Input: dimensioned drawing with shaded views. Units: mm. Origin: part minimum x, y, z. Round coordinates to 2 decimals unless told otherwise and drop trailing zeros. Order: outer loops, then holes, each group sorted by start corner. A loop starts at its lowest first (then second) coordinate and runs counter-clockwise, first axis right, second up. Notation, with made-up numbers: (-8.5, 65) -> (27.5, 65) arc R25 ccw to (27.5, 92) -> close; hole circle Ø2 at (52, 88). An arc over 180 degrees is marked (long way). Use a Markdown table: item, result. Add a question column.
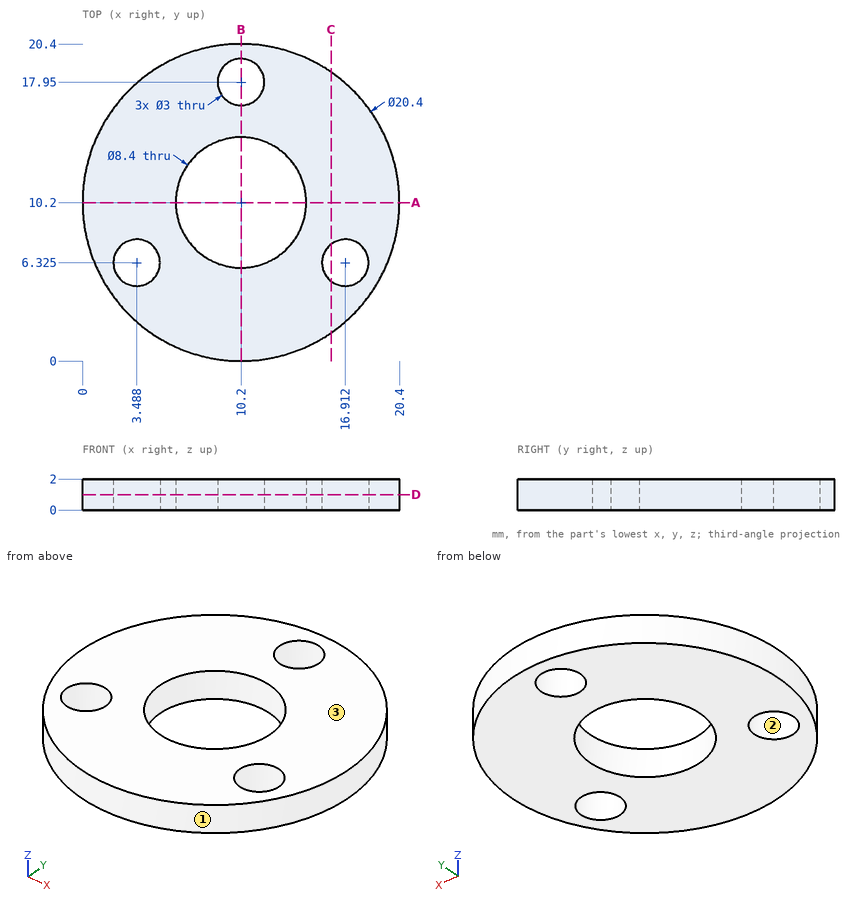
1) Section C-C on x = 16. Output: boundary loops of the cut face in (y, z), then the cut area to 3 significant figures.
2) Line query: probe 1 along Y at (x, z) = (10.2, 1.45); probe 2 along Y at (x, z) = (14, 0.75) (1 decimal); probe 3 along X at (y, z) = (4, 1.1). Output: solid intervals per line, ascending. Write a range as from..to.
3) Section D-D on z = 1. Count the separate pieces of the cut face and the enclosed holes in it, then the cut area to 3 significant figures.
4) Draft query along Y for the marked faces 1, 2 and 3. Return one class per face: pulls with the +Y half, pulls with the -Y half, needs draft (parallel to the pull), parting line crosses it, or undercut.
5) Section B-B on x = 10.2. Output: boundary loops of the cut face in (y, z).
6) First-contact query: pin 1 Ø2.5 at (x, y) = (10.2, 17.95) entering from +Z. Flat tip, straight axial feed; report the tip coordinate or a pass-through.
7) Section A-A on y = 10.2. Output: boundary loops of the cut face in (x, z), then the cut area to 3 significant figures.
Conclusion:
| question | item | result |
|---|---|---|
| 1 | outline | (1.81, 0) -> (5.13, 0) -> (5.13, 2) -> (1.81, 2) -> close; (7.52, 0) -> (18.59, 0) -> (18.59, 2) -> (7.52, 2) -> close |
| 1 | area | 28.8 mm^2 |
| 2 | probe 1 | y = 0..6, 14.4..16.45, 19.45..20.4 |
| 2 | probe 2 | y = 0.7..8.4, 12..19.7 |
| 2 | probe 3 | x = 2.1..18.3 |
| 3 | separate pieces | 1 |
| 3 | enclosed holes | 4 |
| 3 | area | 250 mm^2 |
| 4 | face 1 | parting line crosses it |
| 4 | face 2 | undercut |
| 4 | face 3 | needs draft |
| 5 | outline | (0, 0) -> (6, 0) -> (6, 2) -> (0, 2) -> close; (14.4, 0) -> (16.45, 0) -> (16.45, 2) -> (14.4, 2) -> close; (19.45, 0) -> (20.4, 0) -> (20.4, 2) -> (19.45, 2) -> close |
| 6 | pin 1 | passes through |
| 7 | outline | (0, 0) -> (6, 0) -> (6, 2) -> (0, 2) -> close; (14.4, 0) -> (20.4, 0) -> (20.4, 2) -> (14.4, 2) -> close |
| 7 | area | 24.0 mm^2 |
